Autodesk Inventor part; units mm, degrees
ref_plane "YZ Plane" through (0, 0, 0) normal (1, 0, 0) x (0, 1, 0)
ref_plane "XZ Plane" through (0, 0, 0) normal (0, 1, 0) x (-1, 0, 0)
ref_plane "XY Plane" through (0, 0, 0) normal (0, 0, 1) x (1, 0, 0)
sketch "Sketch1" plane through (0, 0, 0) normal (0, 1, 0) x (-1, 0, 0)
  line L0 (-304.8, 101.6) -> (304.8, 101.6)
  line L1 (304.8, 101.6) -> (304.8, -101.6)
  line L2 (304.8, -101.6) -> (-304.8, -101.6)
  line L3 (-304.8, -101.6) -> (-304.8, 101.6)
  line L4 (-304.8, 101.6) -> (304.8, -101.6) construction
  line L5 (304.8, 101.6) -> (-304.8, -101.6) construction
  point P0 (0, 0)
  dimension "length" = 609.6
  dimension "width" = 203.2
extrude "Extrusion1" add sketch "Sketch1" along normal blind 19.05
sketch "Sketch2" plane through (0, 19.05, 0) normal (0, 1, 0) x (1, 0, 0)
  line L0 (-304.8, -101.6) -> (304.8, -101.6)
  line L1 (304.8, 101.6) -> (-304.8, 101.6)
  line L2 (-304.8, -101.6) -> (-304.8, 101.6)
  line L3 (-304.8, 101.6) -> (-285.75, 101.6)
  line L4 (-285.75, 101.6) -> (-285.75, -101.6)
  line L5 (-285.75, -101.6) -> (-304.8, -101.6)
  point P0 (0, 0)
  dimension "d4" = 19.05
extrude "Extrusion2" add sketch "Sketch2" along normal blind 165.1
ref_plane "Work Plane1" through (0, 0, 101.6) normal (1, 0, 0) x (0, 0, -1)
ref_plane "Work Plane2" through (0, 101.6, 0) normal (0, 1, 0) x (1, 0, 0)
mirror "Mirror1" about plane through (0, 101.6, 0) normal (0, 1, 0) of "Extrusion1"
mirror "Mirror2" about plane through (0, 0, 101.6) normal (1, 0, 0) of "Extrusion2"
equation "\"d4\" = thickness"
properties part number "cabinet" material "Pine, Radiata"
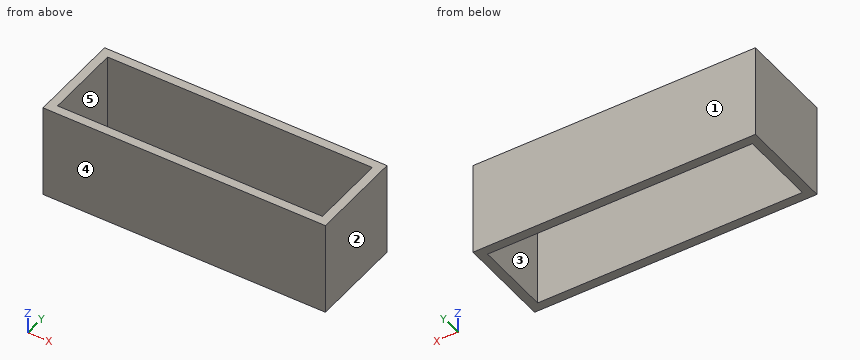
Work out the finished part from the listing and answer in its coordinate system (mm). Face numbers are marked on the shaded views. A direction names the side the tool comes from. Coordinates: 2 decimals unless noted, no trailing zeros. Write each loop counter-clockwise with the first axis right and the second up, starting at its lowest first coordinate (ties: lowest second). Pieces come first, ordered by that corner, then holes. Notation, with made-up numbers: M 11,-10 L 27,-10 A23 ccw 27,26 Z; hole C 7.5,85 d3. An arc over 180 degrees is marked long. Use one line per item in the form item = value. Start each with the question number.
1. The mould has two halves that part along Y. Classify the marked faces 1, 2 and 3: released by +Y, released by -Y, zero draft, split by the parting line, or undercut.
2. The part is cut by section A-A (x = -207). Give the vertices of the cut face in (y, z).
3. Straight lines are drawn through the part: probe 1 along Y at (x, z) = (-209.5, 38); probe 2 along X at (y, z) = (25.5, -83). For each, find the intervals that lie inside material, in ascending order. Write a range as from..to.
4. The part is cut by section B-B (y = 169). Give the vertices of the cut face in (x, z).
5. A tool of negligible diameter and unlimited length cuts with its end or side. For the marked faces 4 and 5, from which of +Z, -Z, +X, -X, +Y, -Y can it reach the whole face along a straight path? Write none if from no direction.
6. The part is cut by section C-C (z = 52). Give the vertices of the cut face in (x, y), plus the area to 3 significant figures.
Evaluation:
q1.face_1 = released by +Y
q1.face_2 = zero draft
q1.face_3 = undercut
q2.outline = M 0,-101.6 L 19.05,-101.6 L 19.05,101.6 L 0,101.6 Z; M 184.15,-101.6 L 203.2,-101.6 L 203.2,101.6 L 184.15,101.6 Z
q3.probe_1 = 0..19.05, 184.15..203.2
q3.probe_2 = -304.8..-285.75, 285.75..304.8
q4.outline = M -304.8,-101.6 L -285.75,-101.6 L -285.75,101.6 L -304.8,101.6 Z; M 285.75,-101.6 L 304.8,-101.6 L 304.8,101.6 L 285.75,101.6 Z
q5.face_4 = +Z, -Z, +X, -X, -Y
q5.face_5 = +Z, -Z
q6.outline = M -304.8,0 L 304.8,0 L 304.8,203.2 L -304.8,203.2 Z; hole M -285.75,19.05 L 285.75,19.05 L 285.75,184.15 L -285.75,184.15 Z
q6.area = 29,500 mm^2
